Check sheet for the modelled part. Datum: model origin and axes. Units: mm. Face numbers are marked on the shaded views. A direction names the side the tool comes from. Coordinates: 2 decimals unless noted, no trailing zeros. Order: outer loops, then holes, each group sorted by start corner. A loop starts at its lowest first (then second) coordinate and runs counter-clockwise, first axis right, second up.
from build123d import *

# Parameters (mm, degrees)
PAD015_DEPTH  = 0.1
SKETCH_W      = 0.9
SKETCH_H      = 10
PAD_DEPTH     = 5
SKETCH024_W   = 0.693804
SKETCH024_H   = 10.010304
SKETCH024_W_2 = 0.997342
SKETCH024_H_2 = 10.046701
POCKET_DEPTH  = 5


with BuildPart() as part:
    # Sketch023 → Pad015 (new body, symmetric)
    with BuildSketch(Plane.YZ):
        Polygon((-26, 1.9), (-26, 1), (-6.9, 1), (-6.9, 0.45), (-14.9, 0.45), (-14.9, -1.9), (-1, -1.9), (-1, -1), (-14, -1), (-14, -0.45), (-6, -0.45), (-6, 1.9), align=None)
    extrude(amount=PAD015_DEPTH, both=True)

    # Sketch (on Face7 of Pad015) → Pad (join)
    with BuildSketch(Plane.ZX.offset(-1)):
        with Locations((-1.45, 5)):
            Rectangle(SKETCH_W, SKETCH_H)
    extrude(amount=PAD_DEPTH)

    # Sketch024 (on Face20 of Pad) → Pocket (cut)
    with BuildSketch(Plane.ZX.offset(4)):
        with Locations((-1.003098, 5.205152)):
            Rectangle(SKETCH024_W, SKETCH024_H)
        with Locations((-2.048671, 5.22335)):
            Rectangle(SKETCH024_W_2, SKETCH024_H_2)
    extrude(amount=-POCKET_DEPTH, mode=Mode.SUBTRACT)


solid = part.part
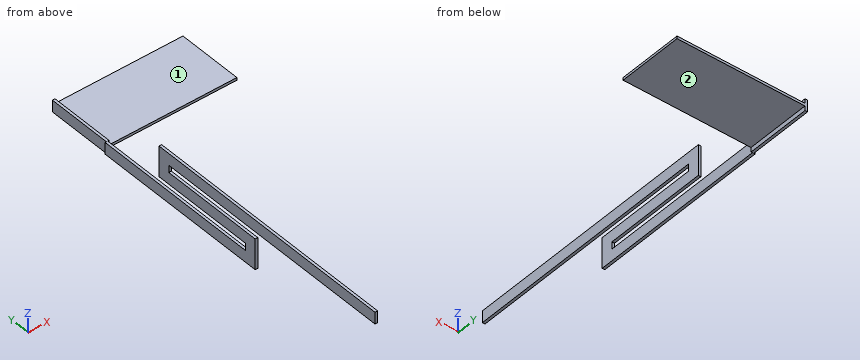
(1) Cross-section at C-C (x = 3). Enter the section's corners in (y, z), and give its area (3 significant figures).
Filled in:
outline: (-1, -1.55) - (4, -1.55) - (4, -1.35) - (-1, -1.35) - close
area: 1.00 mm2
(2) Thickness scan on probe 1 along Z at (x, y) = (9, -0.25); probe 2 along X at (y, z) = (-8.5, -0.15); probe 3 along X at (y, z) = (2.25, -1.25). Record the ranges inside material, lowest first.
Filled in:
probe 1: z = -1.55 to -1.35
probe 2: x = -0.1 to 0.1
probe 3: x = 0 to 0.2
(3) Cross-section at D-D (y = -2.5). Enter the section's corners in (x, z).
Filled in:
outline: (-0.1, -1.9) - (0.1, -1.9) - (0.1, -1) - (-0.1, -1) - close
(4) Cross-section at B-B (y = 1.5). Enter the section's corners in (x, z), and give its area (3 significant figures).
Filled in:
outline: (0, -1.9) - (0.2, -1.9) - (0.2, -1.55) - (10, -1.55) - (10, -1.35) - (0.2, -1.35) - (0.2, -1) - (0, -1) - close
area: 2.14 mm2
(5) Cross-section at A-A (y = -13.5). Enter the section's corners in (x, z), and give its area (3 significant figures).
Filled in:
outline: (-0.1, -1.9) - (0.1, -1.9) - (0.1, -1) - (-0.1, -1) - close; (-0.1, -0.45) - (0.1, -0.45) - (0.1, 0.45) - (-0.1, 0.45) - close; (-0.1, 1) - (0.1, 1) - (0.1, 1.9) - (-0.1, 1.9) - close
area: 0.540 mm2
(6) Tool access check on the marked faces 1 and 2. Record the directions out of +Z, -Z, +X, -X, +Y, -Y that give a thin tool (end or side, any length) a straight path to the whole face; none if there is none.
Filled in:
face 1: +Z, +X, +Y, -Y
face 2: -Z, +X, +Y, -Y
(7) Go/stop test with flat-tipped pins: P1, Ø1, axis at y = 2, z = -1.5, coming from the -X side; P2, Ø4, axis at x = 3.5, y = 1.5, coming from the -Z side; P3, Ø1.5, axis at x = 6, y = 1.5, coming from the +Z side. Record where each tip stops, or that it passes through.
Filled in:
P1: stops at x = 0
P2: stops at z = -1.55
P3: stops at z = -1.35
